Part model, mm, in its own coordinate system. A direction names the side the tool comes from. Round coordinates to 2 decimals unless told otherwise and drop trailing zeros. Loops run counter-clockwise (first coordinate to the right, second up) from the corner with the lowest first, then second, coordinate; pieces in that order, holes last. Notation, with made-up numbers: M 68.5,63 L 96.5,63 A34 ccw 96.5,98 Z; hole C -19,19 d3. An arc over 180 degrees is marked long. Write each question's results on one line, items separated by ' | '.
from build123d import *

# Parameters (mm, degrees)
BOSS_EXTRUDE1_DEPTH     = 60
SKETCH2_R               = 2.5
SKETCH2_R_2             = 19.5
CUT_EXTRUDE1_DEPTH      = 1
CUT_EXTRUDE1_DEPTH_BACK = 61


with BuildPart() as part:
    # Sketch1 → Boss-Extrude1 (new body)
    with BuildSketch(Plane(origin=(0, 0, 0), x_dir=(1, 0, 0), z_dir=(0, 1, 0))):
        Polygon((0, 60), (0, 0), (60, 0), (60, 2), (2, 2), (2, 60), align=None)
    extrude(amount=BOSS_EXTRUDE1_DEPTH)

    # Sketch2 → Cut-Extrude1 (cut, two sides)
    with BuildSketch(Plane.ZY) as cut_extrude1_sk:
        with Locations((-55, 53.55)):
            Circle(SKETCH2_R)
        with Locations((-7.9, 53.55)):
            Circle(SKETCH2_R)
        with Locations((-7.9, 6.45)):
            Circle(SKETCH2_R)
        with Locations((-55, 6.45)):
            Circle(SKETCH2_R)
        with Locations((-31.45, 30)):
            Circle(SKETCH2_R_2)
    extrude(amount=CUT_EXTRUDE1_DEPTH, mode=Mode.SUBTRACT)
    extrude(cut_extrude1_sk.sketch, amount=-CUT_EXTRUDE1_DEPTH_BACK, mode=Mode.SUBTRACT)


solid = part.part
Item 1: Band-saw the part on D-D on y = 53.55. Give the cut face in (x, z).
Filled sheet:
outline: M 0,-60 L 2,-60 L 2,-57.5 L 0,-57.5 Z; M 0,-52.5 L 2,-52.5 L 2,-10.4 L 0,-10.4 Z; M 0,-5.4 L 2,-5.4 L 2,-2 L 60,-2 L 60,0 L 0,0 Z
Item 2: Which spindle directions (+Z, -Z, +X, -X, +Y, -Y) get a long thin tool onto all of the face, cutting with end or side? Do faces 5 (the flat face through (31, 30, -2)), 6 (the cylindrical face through (0.986, 4.929, -9.884)). Say none if no direction does.
Filled sheet:
face 5: -Z, +X, +Y, -Y | face 6: +X, -X
Item 3: Two-plate mould, pull along Y, no slides. Class faces 1 (the cylindrical face through (1, 18.1, -46.9)), 2 (the flat face through (17, 0, -1)), 3 (the flat face through (0, 16, -17)), 4 (the cylindrical face through (0.99, 56.03, -8.23)): +Y half, -Y half, draft (parallel to the pull), parting line (faces both ways), or undercut.
Filled sheet:
face 1: undercut | face 2: -Y half | face 3: draft | face 4: undercut
Item 4: Wall check: L1, parallel to Y at x = 1.4, z = -7.9; L2, parallel to Y at x = 1, z = -7; L3, parallel to Z at x = 1, y = 53. Give the ranges that are in metal, low to high.
Filled sheet:
L1: 0 to 3.95, 8.95 to 51.05, 56.05 to 60 | L2: 0 to 4.12, 8.78 to 51.22, 55.88 to 60 | L3: -60 to -57.44, -52.56 to -10.34, -5.46 to 0
Item 5: Band-saw the part on A-A on z = -55. Give the cut face in (x, y).
Filled sheet:
outline: M 0,0 L 2,0 L 2,3.95 L 0,3.95 Z; M 0,8.95 L 2,8.95 L 2,51.05 L 0,51.05 Z; M 0,56.05 L 2,56.05 L 2,60 L 0,60 Z
Item 6: Band-saw the part on B-B on y = 30. Give the cut face in (x, z).
Filled sheet:
outline: M 0,-60 L 2,-60 L 2,-50.95 L 0,-50.95 Z; M 0,-11.95 L 2,-11.95 L 2,-2 L 60,-2 L 60,0 L 0,0 Z
Item 7: Drop flat-ended pins along their axis: P1, Ø6, axis at y = 53.55, z = -55, coming from the +X side; P2, Ø1.5, axis at x = 14, y = 30.5, coming from the -Z side; P3, Ø12, axis at x = 7.5, z = -48.5, coming from the +Y side. Give the stop position or say it passes through.
Filled sheet:
P1: x = 2 | P2: z = -2 | P3: y = 60
Item 8: Band-saw the part on C-C on z = -34.5. Give the cut face in (x, y).
Filled sheet:
outline: M 0,0 L 2,0 L 2,10.74 L 0,10.74 Z; M 0,49.26 L 2,49.26 L 2,60 L 0,60 Z
